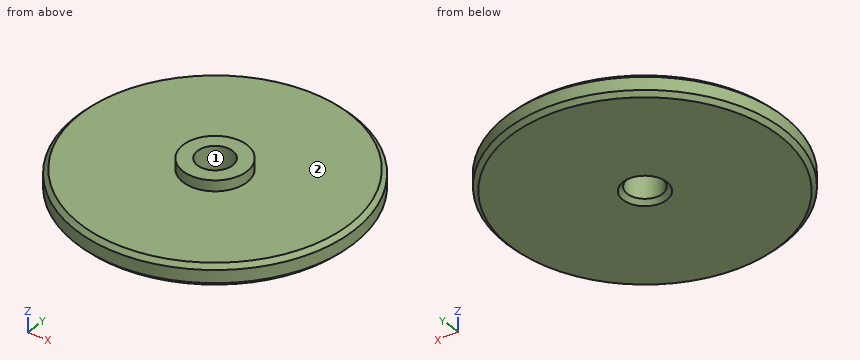
```python
from build123d import *

# Parameters (mm, degrees)
CYLINDER016_R                              = 1.65
CYLINDER016_DEPTH                          = 10
CYLINDER014_R                              = 13
CYLINDER014_DEPTH                          = 2
CYLINDER015_R                              = 3
CYLINDER015_DEPTH                          = 3
CHAMFER004013007011015006009007001083_SIZE = 0.4


with BuildPart() as cylinder016:
    # Cylinder016 → Cylinder016 (new body)
    with BuildSketch(Plane.XY):
        Circle(CYLINDER016_R)
    extrude(amount=CYLINDER016_DEPTH)


with BuildPart() as cylinder014:
    # Cylinder014 → Cylinder014 (new body)
    with BuildSketch(Plane.XY):
        Circle(CYLINDER014_R)
    extrude(amount=CYLINDER014_DEPTH)


with BuildPart() as stopper:
    # Cylinder015 → Cylinder015 (new body)
    with BuildSketch(Plane.XY):
        Circle(CYLINDER015_R)
    extrude(amount=CYLINDER015_DEPTH)

    # Fusion006002011004053036004001028003005014018035002007006011: union Cylinder014
    add(cylinder014.part)

    # Cut008004003004014002002005003004003002003021022001002001106: cut Cylinder016
    add(cylinder016.part, mode=Mode.SUBTRACT)

    # Chamfer004013007011015006009007001083
    chamfer004013007011015006009007001083_edges = [stopper.edges().sort_by_distance(p)[0] for p in [
        (-13, 0, 2),
        (-13, 0, 0),
        (-1.65, 0, 0),
    ]]
    chamfer(chamfer004013007011015006009007001083_edges, length=CHAMFER004013007011015006009007001083_SIZE)


solid = stopper.part
```
Can you work these out from the model? Positions are in its coordinate system, mm. Face numbers are marked on the shaded views. Round coordinates to 2 decimals unless told otherwise and drop trailing zeros. Order: outer loops, then holes, each group sorted by start corner. A loop starts at its lowest first (then second) coordinate and runs counter-clockwise, first axis right, second up.
(1) If I drill on L1, parallel to Y at x = 0, z = 1.2; L2, parallel to Z at x = 4, y = 8; L3, parallel to X at y = -1.5, z = 2.7, over which ranges is the centre line in solid material (lowest first)?
Results are:
L1: y = -13 to -1.65, 1.65 to 13
L2: z = 0 to 2
L3: x = -2.6 to -0.69, 0.69 to 2.6
(2) If we section it at C-C (z = 2.4): Please give me the cut outline in (x, y).
Results are:
outline: circle Ø6 at (0, 0); hole circle Ø3.3 at (0, 0)
(3) I'm going to push flat-ended pins straight in: pin 1 (1.5 mm diameter, centred on y = -4.5, z = 2, fed in from -X); pin 2 (4 mm diameter, centred on x = -2, y = 4.5, fed in from +Z); pin 3 (3 mm diameter, centred on x = -2.5, y = 4.5, fed in from +Z). Where does each tip first touch, or does it pass through?
Results are:
pin 1: stops at x = -12.41
pin 2: stops at z = 3
pin 3: stops at z = 2
(4) If we section it at A-A (y = 0): Please give me the cut outline in (x, z), plus the area to 3 significant figures.
Results are:
outline: (-13, 0.4) - (-12.6, 0) - (-2.05, 0) - (-1.65, 0.4) - (-1.65, 3) - (-3, 3) - (-3, 2) - (-12.6, 2) - (-13, 1.6) - close; (1.65, 0.4) - (2.05, 0) - (12.6, 0) - (13, 0.4) - (13, 1.6) - (12.6, 2) - (3, 2) - (3, 3) - (1.65, 3) - close
area: 47.6 mm2
(5) We'd pull the mould along X, two halves only. Please class the marked faces 1 and 2: +X half, -X half, draft (parallel to the pull), parting line (faces both ways), or undercut.
Results are:
face 1: undercut
face 2: draft
